Check sheet for the modelled part. Datum: model origin and axes. Units: mm. Round coordinates to 2 decimals unless told otherwise and drop trailing zeros. Order: outer loops, then holes, each group sorted by start corner. A loop starts at its lowest first (then second) coordinate and runs counter-clockwise, first axis right, second up.
(1) Thickness scan on probe 1 along Z at (x, y) = (2.5, 1.5); probe 2 along X at (y, z) = (1.1, -37.5); probe 3 along Y at (x, z) = (36, -15). Record the ranges inside material, lowest first.
(2) Sectioned sample at A-A, the plane x = 2.5. Enter the section's corners in (y, z).
(3) Sectioned sample at C-C, the plane x = 37.5. Enter the section's corners in (y, z), and give its area (3 significant figures).
(4) Sectioned sample at D-D, the plane z = -5. Enter the section's corners in (x, y), and give its area (3 significant figures).
(5) Sectioned sample at B-B, the plane z = -37.5. Enter the section's corners in (x, y), and give its area (3 significant figures).
(6) Depth check by flat-ended pin: pin 1 (2.5 mm diameter, centred on x = 2.5, z = -2.5, fed in from +Y); pin 2 (20 mm diameter, centred on x = 10.5, z = -22.5, fed in from +Y); pin 3 (1 mm diameter, centred on x = 30, y = 3, fed in from -Z); pin 4 (0.6 mm diameter, centred on y = 3, z = -5, fed in from -X). Enter the tip coordinate at first touch or a pass-through.
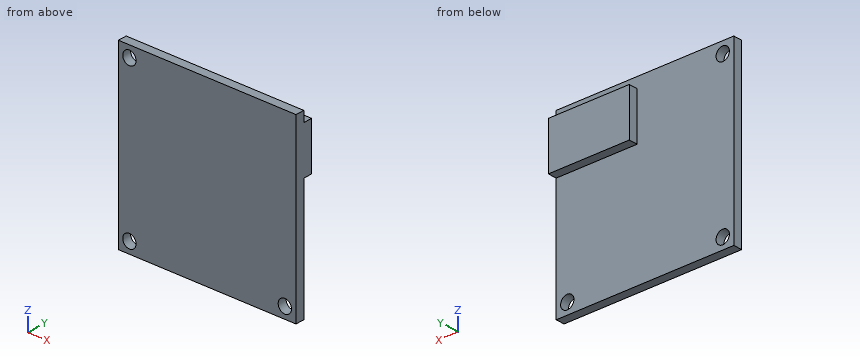
```python
from build123d import *

# Parameters (mm, degrees)
SKETCH1_W           = 40
SKETCH1_H           = 40
BOSS_EXTRUDE1_DEPTH = 2
SKETCH2_R           = 1.5
CUT_EXTRUDE1_DEPTH  = 3
SKETCH3_W           = 18.229825434
SKETCH3_H           = 10.610339614
BOSS_EXTRUDE2_DEPTH = 2


with BuildPart() as part:
    # Sketch1 → Boss-Extrude1 (new body)
    with BuildSketch(Plane(origin=(0, 0, 0), x_dir=(1, 0, 0), z_dir=(0, 1, 0))):
        with Locations((20, 20)):
            Rectangle(SKETCH1_W, SKETCH1_H)
    extrude(amount=BOSS_EXTRUDE1_DEPTH)

    # Sketch2 → Cut-Extrude1 (cut, through all)
    with BuildSketch(Plane(origin=(0, 2, 0), x_dir=(1, 0, 0), z_dir=(0, 1, 0))):
        with Locations((2.5, 37.5)):
            Circle(SKETCH2_R)
        with Locations((37.5, 37.5)):
            Circle(SKETCH2_R)
        with Locations((2.5, 2.5)):
            Circle(SKETCH2_R)
    extrude(amount=-CUT_EXTRUDE1_DEPTH, mode=Mode.SUBTRACT)

    # Sketch3 → Boss-Extrude2 (add)
    with BuildSketch(Plane(origin=(0, 2, 0), x_dir=(1, 0, 0), z_dir=(0, 1, 0))):
        with Locations((30.885087283, 7.630399835)):
            Rectangle(SKETCH3_W, SKETCH3_H)
    extrude(amount=BOSS_EXTRUDE2_DEPTH)


solid = part.part
```
Derived:
1. probe 1: z = -40 to -39, -36 to -4, -1 to 0
1. probe 2: x = 0 to 1, 4 to 36, 39 to 40
1. probe 3: y = 0 to 2
2. outline: (0, -40) - (2, -40) - (2, -39) - (0, -39) - close; (0, -36) - (2, -36) - (2, -4) - (0, -4) - close; (0, -1) - (2, -1) - (2, 0) - (0, 0) - close
3. outline: (0, -40) - (2, -40) - (2, -39) - (0, -39) - close; (0, -36) - (2, -36) - (2, -12.94) - (4, -12.94) - (4, -2.33) - (2, -2.33) - (2, 0) - (0, 0) - close
3. area: 95.2 mm2
4. outline: (0, 0) - (40, 0) - (40, 4) - (21.77, 4) - (21.77, 2) - (0, 2) - close
4. area: 116 mm2
5. outline: (0, 0) - (1, 0) - (1, 2) - (0, 2) - close; (4, 0) - (36, 0) - (36, 2) - (4, 2) - close; (39, 0) - (40, 0) - (40, 2) - (39, 2) - close
5. area: 68.0 mm2
6. pin 1: passes through
6. pin 2: stops at y = 2
6. pin 3: stops at z = -12.94
6. pin 4: stops at x = 21.77
